Input: part model. Units: mm. Frame: model coordinates. A direction names the side the tool comes from. Coordinates: 2 decimals unless noted, no trailing zeros. Write each loop counter-clockwise with the first axis right and the second up, starting at its lowest first coordinate (ties: lowest second). Pieces come first, ordered by that corner, then holes.
from build123d import *

# Parameters (mm, degrees)
SKETCH1_R           = 2.032
BOSS_EXTRUDE1_DEPTH = 1.5875
FILLET1_R           = 19.05


with BuildPart() as part:
    # Sketch1 → Boss-Extrude1 (new, symmetric)
    with BuildSketch(Plane.XY):
        with BuildLine():
            Line((10.998522628, 23.8125), (26.121491242, -2.38125))
            ThreePointArc((26.121491242, -2.38125), (27.390226607, -5.444248127), (27.822968614, -8.73125))
            Line((27.822968614, -8.73125), (27.822968614, -29.239270948))
            Line((27.822968614, -29.239270948), (42.458005799, -48.315226419))
            ThreePointArc((42.458005799, -48.315226419), (44.687348893, -50.145027996), (47.496113055, -50.8))
            Line((47.496113055, -50.8), (47.625, -50.8))
            ThreePointArc((47.625, -50.8), (52.115128061, -48.940128061), (53.975, -44.45))
            Line((53.975, -44.45), (53.975, -12.7))
            ThreePointArc((53.975, -12.7), (53.948566881, -12.198924408), (53.869560945, -11.703411017))
            Line((53.869560945, -11.703411017), (42.458005799, 41.622793369))
            ThreePointArc((42.458005799, 41.622793369), (8.463163904, 49.01990761), (-19.685944915, 28.575))
            Line((-19.685944915, 28.575), (-19.685944915, 15.875))
            ThreePointArc((-19.685944915, 15.875), (-18.273995196, 14.034911301), (-16.131166521, 14.9225))
            Line((-16.131166521, 14.9225), (-10.998522628, 23.8125))
            ThreePointArc((-10.998522628, 23.8125), (0, 30.1625), (10.998522628, 23.8125))
        make_face()
        with Locations((47.625, -44.45)):
            Circle(SKETCH1_R, mode=Mode.SUBTRACT)
        with Locations((49.2125, -12.7)):
            Circle(SKETCH1_R, mode=Mode.SUBTRACT)
    extrude(amount=BOSS_EXTRUDE1_DEPTH, both=True)

    # Fillet1
    fillet1_edges = [part.edges().sort_by_distance(p)[0] for p in [
        (-19.685944915, 28.575, 0),
        (42.458005799, 41.622793369, 0),
    ]]
    fillet(fillet1_edges, radius=FILLET1_R)


solid = part.part
Item 1: Access query for faces 4 (the face through (-18.536, 29.189, -0.022)), 5 (the face through (18.454, 10.899, 0.022)), 6 (the face through (27.823, -19, 0)). Directions: +Z, -Z, +X, -X, +Y, -Y. A direction counts if a zero-diameter tool reaches every point of the face in a straight line with its end or side. Return the directions, or none.
Item 2: Pull-direction query (Y, two-part tool) for faces 1 (the face through (7.105, 48.711, 0.022)), 2 (the face through (47.185, -46.434, -0.022)), 3 (the face through (-13.6, 19.31, 0.02)); classes: released by +Y, released by -Y, zero draft, split by the parting line, or undercut.
Item 3: Section query A-A, the plane z = 1. State how many separate pieces and enclosed holes the cut face has, then the cut area to 3 significant figures.
Item 4: Section query D-D, the plane x = -8. Return loops of the section in (y, z).
Item 5: Section query C-C, the plane y = 18. Return loops of the section in (x, z), then the cut area to 3 significant figures.
Item 6: Pin query (flat end, axial travel): pin 1 Ø3.5 at (x, y) = (47.625, -44.45) entering from -Z. Return the tip coordinate at first contact, or that it passes through.
Item 7: Section query B-B, the plane y = 29. Return loops of the section in (x, z), then the cut area to 3 significant figures.
Item 8: Material intervals for line 1 (X direction, y = -13, z = -0.65) (3 decimals); line 2 (X direction, y = -14, z = 0.8) (3 decimals); line 3 (X direction, y = -23, z = 1.35) (3 decimals), sorted ascending.
The answers:
1. face 4: +Z, -Z, -X, +Y
1. face 5: +Z, -Z, -Y
1. face 6: +Z, -Z, -X, -Y
2. face 1: released by +Y
2. face 2: undercut
2. face 3: released by -Y
3. separate pieces: 1
3. enclosed holes: 2
3. area: 3,150 mm2
4. outline: (27.33, -1.59) - (41.66, -1.59) - (41.66, 1.59) - (27.33, 1.59) - close
5. outline: (-19.69, -1.59) - (-14.35, -1.59) - (-14.35, 1.59) - (-19.69, 1.59) - close; (14.35, -1.59) - (47.51, -1.59) - (47.51, 1.59) - (14.35, 1.59) - close
5. area: 122 mm2
6. pin 1: passes through
7. outline: (-18.6, -1.59) - (-5.31, -1.59) - (-5.31, 1.59) - (-18.6, 1.59) - close; (5.31, -1.59) - (45.16, -1.59) - (45.16, 1.59) - (5.31, 1.59) - close
7. area: 169 mm2
8. line 1: x = 27.823 to 47.203, 51.222 to 53.975
8. line 2: x = 27.823 to 47.651, 50.774 to 53.975
8. line 3: x = 27.823 to 53.975
